Input: part model. Units: mm. Frame: model coordinates. A direction names the side the tool comes from. Round coordinates to 2 decimals unless told otherwise and drop trailing zeros. Loops run counter-clockwise (first coordinate to the right, second up) from the corner with the lowest first, then second, coordinate; pieces in that order, holes last.
(1) Draft query along X for faces 5 (the face through (-41, 10, 3)), 6 (the face through (-37.5, -23, 3)), 7 (the face through (28, -34, 3)). Return one class per face: released by +X, released by -X, zero draft, split by the parting line, or undercut.
(2) Cut plane B-B, the plane z = 4.75. Output: boundary loops of the cut face in (x, y).
(3) Cut plane A-A, the plane y = 32.5. Output: boundary loops of the cut face in (x, z).
(4) Cut plane C-C, the plane y = -25.5. Output: boundary loops of the cut face in (x, z).
(5) Access query for faces 1 (the face through (-27.15, 30.6, 1.48)), 2 (the face through (37.5, 23, 3)), 3 (the face through (37.5, -23, 3)), 4 (the face through (-41, -10, 3)). Directions: +Z, -Z, +X, -X, +Y, -Y. A direction counts if a zero-diameter tool reaches every point of the face in a straight line with its end or side. Return the directions, or none.
(6) First-contact query: pin 1 Ø3.5 at (x, y) = (28.5, 32.5) entering from -Z; pin 2 Ø3 at (x, y) = (28.357, 32.5) entering from +Z; pin 3 Ø2 at (y, z) = (16, 4.5) entering from +X. Flat tips, straight axial feed; report the tip coordinate or a pass-through.
(7) Line query: line 1 (X direction, y = -32.5, z = 4.85); line 2 (X direction, y = -32.5, z = 1.1); line 3 (Y direction, x = 30, z = 0.65). Output: solid intervals per line, ascending.
from build123d import *

# Parameters (mm, degrees)
F0_W     = 6
F0_H     = 20
F1_DEPTH = 6
F2_R     = 2.25
F2_R_2   = 1.143
F3_DEPTH = 3
F4_DEPTH = 6


# Not quite as in the source:
# - a feature names something its author has since deleted; it is built from what else it names


with BuildPart() as f1:
    # F0 (on Top) → F1 (new body)
    with BuildSketch(Plane.XY):
        Polygon((-37.5, -36), (37.5, -36), (37.5, -10), (37.5, 10), (37.5, 36), (-37.5, 36), (-37.5, 10), (-37.5, -10), align=None)
        with Locations((40.5, 0)):
            Rectangle(F0_W, F0_H)
        with Locations((-40.5, 0)):
            Rectangle(F0_W, F0_H)
    extrude(amount=F1_DEPTH)

    # F2 (on face) → F3 (cut)
    with BuildSketch(Plane(origin=(0, 0, 0), x_dir=(1, 0, 0), z_dir=(0, 0, -1))):
        with Locations((-28.357, -32.5)):
            Circle(F2_R)
        with Locations((-28.357, -32.5)):
            Circle(F2_R_2, mode=Mode.SUBTRACT)
        with Locations((28.357, -32.5)):
            Circle(F2_R)
        with Locations((28.357, -32.5)):
            Circle(F2_R_2, mode=Mode.SUBTRACT)
        with Locations((-28.357, 32.5)):
            Circle(F2_R)
        with Locations((-28.357, 32.5)):
            Circle(F2_R_2, mode=Mode.SUBTRACT)
        with Locations((28.357, 32.5)):
            Circle(F2_R)
        with Locations((28.357, 32.5)):
            Circle(F2_R_2, mode=Mode.SUBTRACT)
    extrude(amount=-F3_DEPTH, mode=Mode.SUBTRACT)

    # F2 (on face) → F4 (cut, through all)
    with BuildSketch(Plane(origin=(0, 0, 0), x_dir=(1, 0, 0), z_dir=(0, 0, -1))):
        with Locations((-28.357, -32.5)):
            Circle(F2_R_2)
        with Locations((28.357, -32.5)):
            Circle(F2_R_2)
        with Locations((28.357, 32.5)):
            Circle(F2_R_2)
        with Locations((-28.357, 32.5)):
            Circle(F2_R_2)
    extrude(amount=-F4_DEPTH, mode=Mode.SUBTRACT)


solid = f1.part
Reported:
1. face 5: zero draft
1. face 6: released by -X
1. face 7: undercut
2. outline: (-43.5, -10) - (-37.5, -10) - (-37.5, -36) - (37.5, -36) - (37.5, -10) - (43.5, -10) - (43.5, 10) - (37.5, 10) - (37.5, 36) - (-37.5, 36) - (-37.5, 10) - (-43.5, 10) - close; hole circle Ø2.29 at (-28.36, -32.5); hole circle Ø2.29 at (-28.36, 32.5); hole circle Ø2.29 at (28.36, -32.5); hole circle Ø2.29 at (28.36, 32.5)
3. outline: (-37.5, 0) - (-30.61, 0) - (-30.61, 3) - (-29.5, 3) - (-29.5, 6) - (-37.5, 6) - close; (-27.21, 3) - (-26.11, 3) - (-26.11, 0) - (26.11, 0) - (26.11, 3) - (27.21, 3) - (27.21, 6) - (-27.21, 6) - close; (29.5, 3) - (30.61, 3) - (30.61, 0) - (37.5, 0) - (37.5, 6) - (29.5, 6) - close
4. outline: (-37.5, 0) - (37.5, 0) - (37.5, 6) - (-37.5, 6) - close
5. face 1: -Z
5. face 2: +Z, -Z, +X, +Y
5. face 3: +Z, -Z, +X, -Y
5. face 4: +Z, -Z, -X, -Y
6. pin 1: stops at z = 3
6. pin 2: stops at z = 6
6. pin 3: stops at x = 37.5
7. line 1: x = -37.5 to -29.5, -27.21 to 27.21, 29.5 to 37.5
7. line 2: x = -37.5 to -30.61, -26.11 to 26.11, 30.61 to 37.5
7. line 3: y = -36 to -34.04, -30.96 to 30.96, 34.04 to 36
